Part model, mm, in its own coordinate system. Face numbers are marked on the shaded views. A direction names the side the tool comes from. Coordinates: 2 decimals unless noted, no trailing zeros. Loops run counter-clockwise (first coordinate to the right, second up) from the corner with the lowest first, then second, coordinate; pieces in that order, holes last. Notation, with made-up numbers: (-40, 54) - (-5, 54) arc R17 cw to (-5, 79) - close; hole circle Ø7 at (28, 1). An arc over 180 degrees is marked (long way). Use a Markdown table: item, result. Add a question column.
1) Probe probe 1 along Y at (x, z) = (0, 3.6); probe 2 along Z at (x, y) = (-1.75, 9.25); probe 3 along X at (y, z) = (9.25, 1.5). List the from-to ranges inside material, lowest first. Write a range as [from, to].
2) Band-saw the part on B-B (x = 0). Give the cut face in (y, z), plus the area to 3 significant figures.
3) Band-saw the part on A-A (y = 7). Give the cut face in (x, z).
4) Tool access for the marked faces 4, 5 and 6: list every direction of +Z, -Z, +X, -X, +Y, -Y with a clear straight run to the whole face (end or side of a thin tool).
5) Pull direction X, two halves, no side cores. Call the marked faces 1, 2 and 3: +X half, -X half, draft (parallel to the pull), parting line (faces both ways), or undercut.
6) Band-saw the part on C-C (x = 2). Give the cut face in (y, z).
7) Drop a flat-ended pin along its axis: P1, Ø2, axis at x = -4, y = -4, coming from the +Z side. Give the stop position or say it passes through.
8) Band-saw the part on D-D (z = 2.5). Give the cut face in (x, y), plus the area to 3 significant figures.
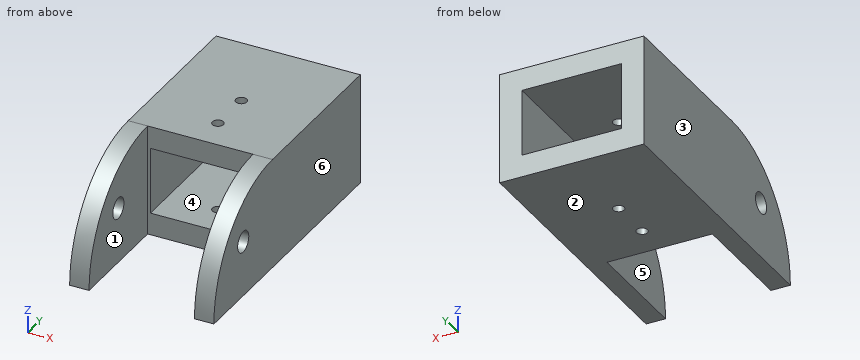
from build123d import *

# Parameters (mm, degrees)
SKETCH1_W               = 13
SKETCH1_H               = 10
SKETCH1_W_2             = 9
SKETCH1_H_2             = 6
BOSS_EXTRUDE1_DEPTH     = 15
BOSS_EXTRUDE2_DEPTH     = 2
SKETCH3_R               = 0.95
CUT_EXTRUDE1_DEPTH      = 14
SKETCH4_R               = 0.5
CUT_EXTRUDE2_DEPTH      = 11
SKETCH5_W               = 0.25
SKETCH5_H               = 10
CUT_EXTRUDE3_DEPTH      = 6
CUT_EXTRUDE3_DEPTH_BACK = 6


with BuildPart() as part:
    # Sketch1 → Boss-Extrude1 (new body)
    with BuildSketch(Plane(origin=(0, 0, 0), x_dir=(1, 0, 0), z_dir=(0, 1, 0))):
        Rectangle(SKETCH1_W, SKETCH1_H)
        Rectangle(SKETCH1_W_2, SKETCH1_H_2, mode=Mode.SUBTRACT)
    extrude(amount=BOSS_EXTRUDE1_DEPTH)

    # Sketch2 → Boss-Extrude2 (add)
    with BuildSketch(Plane(origin=(6.5, 0, 0), x_dir=(0, 0, -1), z_dir=(1, 0, 0))):
        with BuildLine():
            ThreePointArc((-5, 0), (-2.071067812, -7.071067812), (5, -10))
            Line((5, -10), (5, 0))
            Line((5, 0), (-5, 0))
        make_face()
    boss_extrude2 = extrude(amount=-BOSS_EXTRUDE2_DEPTH)

    # Mirror1: Boss-Extrude2 across plane
    add(boss_extrude2.mirror(Plane(origin=(0, 0, 0), x_dir=(0, 0, 1), z_dir=(1, 0, 0))))

    # Sketch3 → Cut-Extrude1 (cut, through all)
    with BuildSketch(Plane(origin=(6.5, 0, 0), x_dir=(0, 0, -1), z_dir=(1, 0, 0))):
        with Locations((0, -5)):
            Circle(SKETCH3_R)
    extrude(amount=-CUT_EXTRUDE1_DEPTH, mode=Mode.SUBTRACT)

    # Sketch4 → Cut-Extrude2 (cut, through all)
    with BuildSketch(Plane.XY.offset(5)):
        with Locations((0, 3)):
            Circle(SKETCH4_R)
        with Locations((0, 7)):
            Circle(SKETCH4_R)
    extrude(amount=-CUT_EXTRUDE2_DEPTH, mode=Mode.SUBTRACT)

    # Sketch5 → Cut-Extrude3 (cut, two sides)
    with BuildSketch(Plane.XY) as cut_extrude3_sk:
        with Locations((-4.625, -5)):
            Rectangle(SKETCH5_W, SKETCH5_H)
        with Locations((4.625, -5)):
            Rectangle(SKETCH5_W, SKETCH5_H)
    extrude(amount=CUT_EXTRUDE3_DEPTH, mode=Mode.SUBTRACT)
    extrude(cut_extrude3_sk.sketch, amount=-CUT_EXTRUDE3_DEPTH_BACK, mode=Mode.SUBTRACT)


solid = part.part
Answer block:
| question | item | result |
|---|---|---|
| 1 | probe 1 | [0, 2.5], [3.5, 6.5], [7.5, 15] |
| 1 | probe 2 | [-5, -3], [3, 5] |
| 1 | probe 3 | [-6.5, -4.5], [4.5, 6.5] |
| 2 | outline | (0, -5) - (2.5, -5) - (2.5, -3) - (0, -3) - close; (0, 3) - (2.5, 3) - (2.5, 5) - (0, 5) - close; (3.5, -5) - (6.5, -5) - (6.5, -3) - (3.5, -3) - close; (3.5, 3) - (6.5, 3) - (6.5, 5) - (3.5, 5) - close; (7.5, -5) - (15, -5) - (15, -3) - (7.5, -3) - close; (7.5, 3) - (15, 3) - (15, 5) - (7.5, 5) - close |
| 2 | area | 52.0 mm2 |
| 3 | outline | (-6.5, -5) - (-0.5, -5) - (-0.5, -3) - (-4.5, -3) - (-4.5, 3) - (-0.5, 3) - (-0.5, 5) - (-6.5, 5) - close; (0.5, -5) - (6.5, -5) - (6.5, 5) - (0.5, 5) - (0.5, 3) - (4.5, 3) - (4.5, -3) - (0.5, -3) - close |
| 4 | face 4 | +Y, -Y |
| 4 | face 5 | +Z, -Z, -Y |
| 4 | face 6 | +Z, -Z, +X, +Y, -Y |
| 5 | face 1 | undercut |
| 5 | face 2 | draft |
| 5 | face 3 | -X half |
| 6 | outline | (0, -5) - (15, -5) - (15, -3) - (0, -3) - close; (0, 3) - (15, 3) - (15, 5) - (0, 5) - close |
| 7 | P1 | z = 4.43 |
| 8 | outline | (-6.5, -6.61) - (-4.75, -6.61) - (-4.75, 0) - (-4.5, 0) - (-4.5, 15) - (-6.5, 15) - close; (4.5, 0) - (4.75, 0) - (4.75, -6.61) - (6.5, -6.61) - (6.5, 15) - (4.5, 15) - close |
| 8 | area | 83.2 mm2 |
